Geometry check sheet. Reference: the model listing, model coordinates, mm. A direction names the side the tool comes from. Round coordinates to 2 decimals unless told otherwise and drop trailing zeros. Write each loop counter-clockwise with the first axis right and the second up, starting at its lowest first coordinate (ties: lowest second). Pieces come first, ordered by that corner, then holes. Notation, with made-up numbers: M 72,6 L 78,6 A16 ccw 78,35 Z; hole C 46.25,69 d9. An arc over 180 degrees is marked long. One line per item, written item: value. Start each with the question number.
1. Section check D-D (z = -0.25). Record the boundary of the cut face in (x, y), and give its area (3 significant figures).
2. Release check for a two-part mould opening along Y. For faces 6 (the flat face through (4, 4.762, 3)), 7 (the flat face through (7.938, -1, 0)), 8 (the cylindrical face through (5.16, -5.21, -1.97)) record: pulls with the +Y half, pulls with the -Y half, needs draft (parallel to the pull), parting line crosses it, or undercut.
3. Section check A-A (y = 0.5). Record the boundary of the cut face in (x, z), and give its area (3 significant figures).
4. Section check B-B (z = -2.75). Record the boundary of the cut face in (x, y), and give its area (3 significant figures).
5. Scan lines: probe 1 along Y at (x, z) = (4, 1); probe 2 along Y at (x, z) = (4, 4.5); probe 3 along Y at (x, z) = (1, 1.5). Record each from-to range of solid material in increasing order. Write a range as [from, to].
6. Section check C-C (y = 3.75). Record the boundary of the cut face in (x, z).
7. Depth check by flat-ended pin: P1, Ø2.5, axis at x = 3.5, y = 2.5, coming from the -Z side; P2, Ø1.2, axis at x = 4, y = -5, coming from the -Z side; P3, Ø0.9, axis at x = 7.5, z = -3, coming from the -Y side; P4, Ø8, axis at y = 2, z = -4, coming from the -X side. Enter the tip coordinate at first touch or a pass-through.
8. Access from +Z, -Z, +X, -X, +Y, -Y to the whole of each face (thin tool, end or side, straight path). Record for faces 1 (the flat face through (4, -5, -3.969)), 2 (the flat face through (3, -4, 0.794)), 3 (the cylindrical face through (4.01, -1.19, -3.92)), 4 (the cylindrical face through (5.63, 2.41, 5.7)), 5 (the cylindrical face through (2.48, 2.41, -2.89)).
from build123d import *

# Parameters (mm, degrees)
SKETCH1_W           = 7.9375
SKETCH1_H           = 2.38125
BOSS_EXTRUDE1_DEPTH = 7.14375
SKETCH2_R           = 3.96875
BOSS_EXTRUDE2_DEPTH = 0.79375
SKETCH3_R           = 3.96875
CUT_EXTRUDE1_DEPTH  = 14.661957117
SKETCH4_W           = 4.7625
SKETCH4_H           = 4.7625
BOSS_EXTRUDE3_DEPTH = 4.7625
SKETCH5_R           = 1.27
SKETCH5_R_2         = 1.190625
CUT_EXTRUDE2_DEPTH  = 4.7625
CUT_EXTRUDE3_DEPTH  = 14.216592983
SKETCH7_R           = 1.190625
BOSS_EXTRUDE4_DEPTH = 2.38125
SKETCH8_R           = 0.9921875
BOSS_EXTRUDE5_DEPTH = 0.79375
SKETCH9_W           = 2.032
SKETCH9_H           = 0.79375
CUT_EXTRUDE4_DEPTH  = 0.79375


with BuildPart() as part:
    # Sketch1 → Boss-Extrude1 (new body)
    with BuildSketch(Plane.XY):
        with Locations((3.96875, -1.190625)):
            Rectangle(SKETCH1_W, SKETCH1_H)
    boss_extrude1 = extrude(amount=BOSS_EXTRUDE1_DEPTH)

    # Sketch2 → Boss-Extrude2 (add)
    with BuildSketch(Plane(origin=(0, 0, 0), x_dir=(-1, 0, 0), z_dir=(0, 0, -1))):
        with Locations((-3.96875, -5.159375)):
            Circle(SKETCH2_R)
    boss_extrude2 = extrude(amount=-BOSS_EXTRUDE2_DEPTH)

    # Sketch3 → Cut-Extrude1 (cut, through all)
    with BuildSketch(Plane.XY.offset(0.79375)):
        with Locations((3.96875, -5.159375)):
            Circle(SKETCH3_R)
    cut_extrude1 = extrude(amount=CUT_EXTRUDE1_DEPTH, mode=Mode.SUBTRACT)

    # Sketch4 → Boss-Extrude3 (add)
    with BuildSketch(Plane(origin=(0, 0, 0), x_dir=(1, 0, 0), z_dir=(0, 1, 0))):
        with Locations((3.96875, -4.365625)):
            Rectangle(SKETCH4_W, SKETCH4_H)
    boss_extrude3 = extrude(amount=BOSS_EXTRUDE3_DEPTH)

    # Sketch5 → Cut-Extrude2 (cut)
    with BuildSketch(Plane(origin=(0, 4.7625, 0), x_dir=(1, 0, 0), z_dir=(0, 1, 0))):
        with Locations((1.5875, -6.746875)):
            Circle(SKETCH5_R)
        with Locations((1.5875, -1.984375)):
            Circle(SKETCH5_R)
        with Locations((6.35, -1.984375)):
            Circle(SKETCH5_R)
        with Locations((6.35, -6.746875)):
            Circle(SKETCH5_R)
        with Locations(Location((3.96875, -4.365625, 0), (0, 0, 270))):
            Circle(SKETCH5_R_2)
    cut_extrude2 = extrude(amount=-CUT_EXTRUDE2_DEPTH, mode=Mode.SUBTRACT)

    # Sketch6 → Cut-Extrude3 (cut, through all)
    with BuildSketch(Plane.ZY.offset(-1.5875)):
        Polygon((6.746875, 0.6985), (6.746875, 5.7785), (5.730875, 5.7785), align=None)
    cut_extrude3 = extrude(amount=-CUT_EXTRUDE3_DEPTH, mode=Mode.SUBTRACT)

    # Sketch7 → Boss-Extrude4 (add)
    with BuildSketch(Plane.XY.offset(0.79375)):
        with Locations(Location((3.96875, -5.159375, 0), (0, 0, 180))):
            Circle(SKETCH7_R)
    boss_extrude4 = extrude(amount=BOSS_EXTRUDE4_DEPTH)

    # Sketch8 → Boss-Extrude5 (add)
    with BuildSketch(Plane.XY.offset(3.175)):
        with Locations((3.96875, -5.159375)):
            Circle(SKETCH8_R)
    boss_extrude5 = extrude(amount=BOSS_EXTRUDE5_DEPTH)

    # Sketch9 → Cut-Extrude4 (cut)
    with BuildSketch(Plane.XY.offset(3.96875)):
        with Locations((3.96875, -4.365625)):
            Rectangle(SKETCH9_W, SKETCH9_H)
    cut_extrude4 = extrude(amount=-CUT_EXTRUDE4_DEPTH, mode=Mode.SUBTRACT)

    # Mirror1: Boss-Extrude1, Boss-Extrude2, Cut-Extrude1, Boss-Extrude3, Cut-Extrude2, Cut-Extrude3, Boss-Extrude4, Boss-Extrude5, Cut-Extrude4 across plane
    add(boss_extrude1.mirror(Plane.XY))
    add(boss_extrude2.mirror(Plane.XY))
    add(cut_extrude1.mirror(Plane.XY), mode=Mode.SUBTRACT)
    add(boss_extrude3.mirror(Plane.XY))
    add(cut_extrude2.mirror(Plane.XY), mode=Mode.SUBTRACT)
    add(cut_extrude3.mirror(Plane.XY), mode=Mode.SUBTRACT)
    add(boss_extrude4.mirror(Plane.XY))
    add(boss_extrude5.mirror(Plane.XY))
    add(cut_extrude4.mirror(Plane.XY), mode=Mode.SUBTRACT)


solid = part.part
Result sheet:
1. outline: M 0,-2.38 L 1.13,-2.38 A3.97 ccw long 6.8,-2.38 L 7.94,-2.38 L 7.94,0 L 0,0 Z
1. area: 63.7 mm2
2. face 6: pulls with the +Y half
2. face 7: needs draft
2. face 8: undercut
3. outline: M 1.59,-5.48 A1.27 cw 2.86,-6.75 L 5.08,-6.75 A1.27 cw 6.35,-5.48 L 6.35,-3.25 A1.27 cw 5.08,-1.98 L 2.86,-1.98 A1.27 cw 1.59,-3.25 Z; M 1.59,3.25 A1.27 cw 2.86,1.98 L 5.08,1.98 A1.27 cw 6.35,3.25 L 6.35,5.48 A1.27 cw 5.08,6.75 L 2.86,6.75 A1.27 cw 1.59,5.48 Z; hole C 3.97,-4.37 d2.38; hole C 3.97,4.37 d2.38
3. area: 26.3 mm2
4. outline: M 0,-2.38 L 1.13,-2.38 A3.97 cw 6.8,-2.38 L 7.94,-2.38 L 7.94,0 L 5.34,0 L 5.34,4.76 L 2.6,4.76 L 2.6,0 L 0,0 Z; C 3.97,-5.16 d2.38
4. area: 31.7 mm2
5. probe 1: y = [-6.35, -3.97], [-1.19, 0]
5. probe 2: y = [-1.19, 0]
5. probe 3: y = [-2.38, 0]
6. outline: M 1.59,-5.48 A1.27 cw 2.7,-6.14 L 5.24,-6.14 A1.27 cw 6.35,-5.48 L 6.35,-3.25 A1.27 cw 5.08,-1.98 L 2.86,-1.98 A1.27 cw 1.59,-3.25 Z; M 1.59,3.25 A1.27 cw 2.86,1.98 L 5.08,1.98 A1.27 cw 6.35,3.25 L 6.35,5.48 A1.27 cw 5.24,6.14 L 2.7,6.14 A1.27 cw 1.59,5.48 Z; hole C 3.97,-4.37 d2.38; hole C 3.97,4.37 d2.38
7. P1: stops at z = -6.64
7. P2: stops at z = -3.97
7. P3: stops at y = -2.38
7. P4: stops at x = 0
8. face 1: -Z, +X, -X, -Y
8. face 2: +Z
8. face 3: -Z
8. face 4: +Z, +X, +Y
8. face 5: -X, +Y
